from build123d import *

# Parameters (mm, degrees)
SKETCH_1_W               = 127.3
SKETCH_1_H               = 127.3
EXTRUDE_1_DEPTH          = 16.25
SKETCH_2_W               = 8.5
SKETCH_2_H               = 8.5
EXTRUDE_2_DEPTH          = 0.5
SKETCH_3_R               = 6
EXTRUDE_3_DEPTH          = 6
MIRROR_2_COPY_1_SKETCH_R = 6
MIRROR_2_COPY_1_DEPTH    = 6
SKETCH_4_R               = 3.25
CUT_EXTRUDE_1_DEPTH      = 3
MIRROR_4_COPY_1_SKETCH_R = 3.25
MIRROR_4_COPY_1_DEPTH    = 3
FILLET_1_R               = 10
SKETCH_5_R               = 1.6
CUT_EXTRUDE_2_DEPTH      = 3


with BuildPart() as part:
    # 草图1 → 凸台-拉伸1 (new, symmetric)
    with BuildSketch(Plane(origin=(0, 0, 0), x_dir=(1, 0, 0), z_dir=(0, 1, 0))):
        Rectangle(SKETCH_1_W, SKETCH_1_H)
    extrude(amount=EXTRUDE_1_DEPTH, both=True)

    # 草图2 → 凸台-拉伸2 (add, symmetric)
    with BuildSketch(Plane.XY.offset(63.65)):
        with Locations((41.9, -2.5)):
            Rectangle(SKETCH_2_W, SKETCH_2_H)
    extrude(amount=EXTRUDE_2_DEPTH, both=True)

    # 草图3 → 凸台-拉伸3 (add)
    with BuildSketch(Plane.XZ.offset(16.25)):
        with Locations(Location((51.65, 51.65, 0), (0, 0, 90))):
            Circle(SKETCH_3_R)
    extrude_3 = extrude(amount=EXTRUDE_3_DEPTH)

    # 镜向1: 凸台-拉伸3 across plane
    add(extrude_3.mirror(Plane.XY))

    # 镜向2: 凸台-拉伸3 across plane
    add(extrude_3.mirror(Plane(origin=(0, 0, 0), x_dir=(0, 0, 1), z_dir=(1, 0, 0))))

    # 镜向2 copy 1 sketch → 镜向2 copy 1 (add)
    with BuildSketch(Plane(origin=(0, -16.25, 0), x_dir=(-1, 0, 0), z_dir=(0, -1, 0))):
        with Locations(Location((51.65, 51.65, 0), (0, 0, 90))):
            Circle(MIRROR_2_COPY_1_SKETCH_R)
    extrude(amount=MIRROR_2_COPY_1_DEPTH)

    # 草图4 → 切除-拉伸1 (cut)
    with BuildSketch(Plane(origin=(0, 16.25, 0), x_dir=(1, 0, 0), z_dir=(0, 1, 0))):
        with Locations(Location((56, 49.5, 0), (0, 0, 270))):
            Circle(SKETCH_4_R)
    cut_extrude_1 = extrude(amount=-CUT_EXTRUDE_1_DEPTH, mode=Mode.SUBTRACT)

    # 镜向3: 切除-拉伸1 across plane
    add(cut_extrude_1.mirror(Plane(origin=(0, 0, 0), x_dir=(0, 0, 1), z_dir=(1, 0, 0))), mode=Mode.SUBTRACT)

    # 镜向4: 切除-拉伸1 across plane
    add(cut_extrude_1.mirror(Plane.XY), mode=Mode.SUBTRACT)

    # 镜向4 copy 1 sketch → 镜向4 copy 1 (cut)
    with BuildSketch(Plane(origin=(0, 16.25, 0), x_dir=(-1, 0, 0), z_dir=(0, 1, 0))):
        with Locations(Location((56, 49.5, 0), (0, 0, 270))):
            Circle(MIRROR_4_COPY_1_SKETCH_R)
    extrude(amount=-MIRROR_4_COPY_1_DEPTH, mode=Mode.SUBTRACT)

    # 圆角1
    fillet_1_edges = [part.edges().sort_by_distance(p)[0] for p in [
        (63.65, 0, 63.65),
        (-63.65, 0, 63.65),
        (-63.65, 0, -63.65),
        (63.65, 0, -63.65),
    ]]
    fillet(fillet_1_edges, radius=FILLET_1_R)

    # 草图5 → 切除-拉伸2 (cut)
    with BuildSketch(Plane.XZ.offset(16.25)):
        with Locations(Location((-48, 0, 0), (0, 0, 270))):
            Circle(SKETCH_5_R)
        with Locations(Location((48, 0, 0), (0, 0, 270))):
            Circle(SKETCH_5_R)
    extrude(amount=-CUT_EXTRUDE_2_DEPTH, mode=Mode.SUBTRACT)


solid = part.part
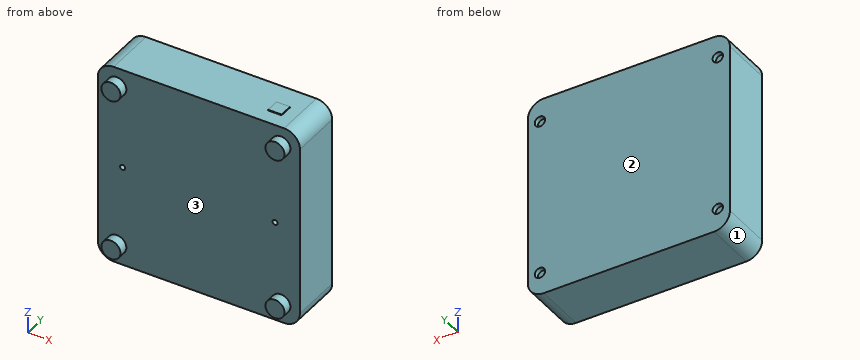
Work out the finished part from the listing and answer in its coordinate system (mm). Face numbers are marked on the shaded views. Give positions to 0.01 mm unless a question says otherwise; leave off trailing zeros. Write each loop counter-clockwise with the first axis right and the second up, starting at its lowest first coordinate (ties: lowest second). Pieces come first, ordered by that corner, then holes.
Q1. The part is cut by section A-A on x = 42. Give the vertices of the cut face in (y, z), and give its area (3 significant figures).
Answer:
outline: (-16.25, -63.65) - (16.25, -63.65) - (16.25, 63.65) - (1.75, 63.65) - (1.75, 64.15) - (-6.75, 64.15) - (-6.75, 63.65) - (-16.25, 63.65) - close
area: 4,140 mm2
Q2. The part is cut by section C-C on x = -56. Give the vertices of the cut face in (y, z).
Answer:
outline: (-22.25, -55.78) - (-16.25, -55.78) - (-16.25, -63.37) - (16.25, -63.37) - (16.25, -52.75) - (13.25, -52.75) - (13.25, -46.25) - (16.25, -46.25) - (16.25, 46.25) - (13.25, 46.25) - (13.25, 52.75) - (16.25, 52.75) - (16.25, 63.37) - (-16.25, 63.37) - (-16.25, 55.78) - (-22.25, 55.78) - (-22.25, 47.52) - (-16.25, 47.52) - (-16.25, -47.52) - (-22.25, -47.52) - close
Q3. Given pin 1 (6 mm diameter, centred on x = 56, z = -49.5, fed in from +Y); pin 2 (2.5 mm diameter, centred on x = -47.5, z = -0.5, fed in from -Y); pin 3 (1 mm diameter, centred on x = 48.5, z = 0.5, fed in from -Y), each flat-ended and moving along its own axis, determine where each tip first touches the part or whether it passes through.
Answer:
pin 1: stops at y = 13.25
pin 2: stops at y = -16.25
pin 3: stops at y = -13.25
Q4. For a pull along Z with two mould halves and no side action, classify the marked faces 1, 2 and 3 as released by +Z, released by -Z, zero draft, split by the parting line, or undercut.
Answer:
face 1: released by -Z
face 2: zero draft
face 3: undercut
Q5. The part is cut by section B-B on z = 49.5. Give the vertices of the cut face in (x, y), and give its area (3 significant figures).
Answer:
outline: (-63.65, -16.25) - (-57.25, -16.25) - (-57.25, -22.25) - (-46.05, -22.25) - (-46.05, -16.25) - (46.05, -16.25) - (46.05, -22.25) - (57.25, -22.25) - (57.25, -16.25) - (63.65, -16.25) - (63.65, 16.25) - (59.25, 16.25) - (59.25, 13.25) - (52.75, 13.25) - (52.75, 16.25) - (-52.75, 16.25) - (-52.75, 13.25) - (-59.25, 13.25) - (-59.25, 16.25) - (-63.65, 16.25) - close
area: 4,230 mm2
Q6. The part is cut by section D-D on z = -29. Give the vertices of the cut face in (x, y).
Answer:
outline: (-63.65, -16.25) - (63.65, -16.25) - (63.65, 16.25) - (-63.65, 16.25) - close
Q7. Straight lines are drawn through the part: L1, parallel to X at y = -14.7, z = 0; L2, parallel to Z at x = -56, y = 15.35; L3, parallel to X at y = 15, z = 49. For each, find the intervals that lie inside material, in ascending order.
Answer:
L1: x = -63.65 to -49.6, -46.4 to 46.4, 49.6 to 63.65
L2: z = -63.37 to -52.75, -46.25 to 46.25, 52.75 to 63.37
L3: x = -63.65 to -59.21, -52.79 to 52.79, 59.21 to 63.65
